CAD build for the part. Positions are in the model's coordinates, mm. Give positions to 0.01 mm unless a question says otherwise; leave off trailing zeros. Write each loop counter-clockwise with the first axis right and the second up, starting at its lowest first coordinate (ties: lowest second). Pieces come first, ordered by that corner, then holes. Notation, with made-up numbers: (80, 12.25) -> (104, 12.25) arc R25 cw to (104, 30.25) -> close; hole circle Ø5 at (67.5, 27.5). An arc over 180 degrees is marked (long way). Use one line per item in the form item = value. Start each with the question number.
from build123d import *

# Parameters (mm, degrees)
SKETCH1_W           = 105
SKETCH1_H           = 105
SKETCH1_W_2         = 3
SKETCH1_H_2         = 3.682816402
SKETCH1_W_3         = 3.682816402
SKETCH1_H_3         = 3
BOSS_EXTRUDE1_DEPTH = 3


with BuildPart() as part:
    # Sketch1 → Boss-Extrude1 (new body)
    with BuildSketch(Plane.XY):
        with Locations((55.5, 244.5)):
            Rectangle(SKETCH1_W, SKETCH1_H)
        with Locations((19.5, 240.958607901)):
            Rectangle(SKETCH1_W_2, SKETCH1_H_2, mode=Mode.SUBTRACT)
        with Locations((7.5, 240.958607901)):
            Rectangle(SKETCH1_W_2, SKETCH1_H_2, mode=Mode.SUBTRACT)
        with Locations((31.5, 240.958607901)):
            Rectangle(SKETCH1_W_2, SKETCH1_H_2, mode=Mode.SUBTRACT)
        with Locations((51.958607901, 232.5)):
            Rectangle(SKETCH1_W_3, SKETCH1_H_3, mode=Mode.SUBTRACT)
        with Locations((51.958607901, 220.5)):
            Rectangle(SKETCH1_W_3, SKETCH1_H_3, mode=Mode.SUBTRACT)
        with Locations((51.958607901, 280.5)):
            Rectangle(SKETCH1_W_3, SKETCH1_H_3, mode=Mode.SUBTRACT)
        with Locations((51.958607901, 268.5)):
            Rectangle(SKETCH1_W_3, SKETCH1_H_3, mode=Mode.SUBTRACT)
        with Locations((79.5, 240.958607901)):
            Rectangle(SKETCH1_W_2, SKETCH1_H_2, mode=Mode.SUBTRACT)
        with Locations((91.5, 240.958607901)):
            Rectangle(SKETCH1_W_2, SKETCH1_H_2, mode=Mode.SUBTRACT)
        with Locations((51.958607901, 292.5)):
            Rectangle(SKETCH1_W_3, SKETCH1_H_3, mode=Mode.SUBTRACT)
        with Locations((7.5, 248.041392099)):
            Rectangle(SKETCH1_W_2, SKETCH1_H_2, mode=Mode.SUBTRACT)
        with Locations((19.5, 248.041392099)):
            Rectangle(SKETCH1_W_2, SKETCH1_H_2, mode=Mode.SUBTRACT)
        with Locations((31.5, 248.041392099)):
            Rectangle(SKETCH1_W_2, SKETCH1_H_2, mode=Mode.SUBTRACT)
        with Locations((67.5, 248.041392099)):
            Rectangle(SKETCH1_W_2, SKETCH1_H_2, mode=Mode.SUBTRACT)
        with Locations((43.5, 248.041392099)):
            Rectangle(SKETCH1_W_2, SKETCH1_H_2, mode=Mode.SUBTRACT)
        with Locations((79.5, 248.041392099)):
            Rectangle(SKETCH1_W_2, SKETCH1_H_2, mode=Mode.SUBTRACT)
        with Locations((91.5, 248.041392099)):
            Rectangle(SKETCH1_W_2, SKETCH1_H_2, mode=Mode.SUBTRACT)
        with Locations((103.5, 248.041392099)):
            Rectangle(SKETCH1_W_2, SKETCH1_H_2, mode=Mode.SUBTRACT)
        with Locations((43.5, 240.958607901)):
            Rectangle(SKETCH1_W_2, SKETCH1_H_2, mode=Mode.SUBTRACT)
        with Locations((67.5, 240.958607901)):
            Rectangle(SKETCH1_W_2, SKETCH1_H_2, mode=Mode.SUBTRACT)
        with Locations((103.5, 240.958607901)):
            Rectangle(SKETCH1_W_2, SKETCH1_H_2, mode=Mode.SUBTRACT)
        with Locations((59.041392099, 292.5)):
            Rectangle(SKETCH1_W_3, SKETCH1_H_3, mode=Mode.SUBTRACT)
        with Locations((59.041392099, 280.5)):
            Rectangle(SKETCH1_W_3, SKETCH1_H_3, mode=Mode.SUBTRACT)
        with Locations((59.041392099, 268.5)):
            Rectangle(SKETCH1_W_3, SKETCH1_H_3, mode=Mode.SUBTRACT)
        with Locations((59.041392099, 256.5)):
            Rectangle(SKETCH1_W_3, SKETCH1_H_3, mode=Mode.SUBTRACT)
        with Locations((59.041392099, 244.5)):
            Rectangle(SKETCH1_W_3, SKETCH1_H_3, mode=Mode.SUBTRACT)
        with Locations((59.041392099, 232.5)):
            Rectangle(SKETCH1_W_3, SKETCH1_H_3, mode=Mode.SUBTRACT)
        with Locations((59.041392099, 220.5)):
            Rectangle(SKETCH1_W_3, SKETCH1_H_3, mode=Mode.SUBTRACT)
        with Locations((59.041392099, 208.5)):
            Rectangle(SKETCH1_W_3, SKETCH1_H_3, mode=Mode.SUBTRACT)
        with Locations((59.041392099, 196.5)):
            Rectangle(SKETCH1_W_3, SKETCH1_H_3, mode=Mode.SUBTRACT)
        with Locations((51.958607901, 244.5)):
            Rectangle(SKETCH1_W_3, SKETCH1_H_3, mode=Mode.SUBTRACT)
        with Locations((51.958607901, 256.5)):
            Rectangle(SKETCH1_W_3, SKETCH1_H_3, mode=Mode.SUBTRACT)
        with Locations((51.958607901, 196.5)):
            Rectangle(SKETCH1_W_3, SKETCH1_H_3, mode=Mode.SUBTRACT)
        with Locations((51.958607901, 208.5)):
            Rectangle(SKETCH1_W_3, SKETCH1_H_3, mode=Mode.SUBTRACT)
    extrude(amount=BOSS_EXTRUDE1_DEPTH)


solid = part.part
1) Wall check: line 1 along Y through (x, z) = (31, 2.1); line 2 along X through (y, z) = (281, 0.5). Give the ranges that are in metal, low to high. Write a range as from..to.
2) Cut at A-A (x = 91.5). Give the cut face in (y, z), and give its area (3 significant figures).
3) Cut at B-B (z = 0.6). State how many separate pieces and enclosed holes the cut face has, and give its area (3 significant figures).
Final values:
q1.line_1 = 192..239.12, 242.8..246.2, 249.88..297
q1.line_2 = 3..50.12, 53.8..57.2, 60.88..108
q2.outline = (192, 0) -> (239.12, 0) -> (239.12, 3) -> (192, 3) -> close; (242.8, 0) -> (246.2, 0) -> (246.2, 3) -> (242.8, 3) -> close; (249.88, 0) -> (297, 0) -> (297, 3) -> (249.88, 3) -> close
q2.area = 293 mm^2
q3.separate_pieces = 1
q3.enclosed_holes = 34
q3.area = 10,600 mm^2
